The listing builds one solid part. Answer for the finished solid, in the listing's coordinates (mm). A direction names the side the tool comes from. Give positions to 0.01 mm unless a question says otherwise; leave off trailing zeros. Order: outer loops, then holes, each group sorted by start corner. A loop starts at its lowest first (then second) coordinate and runs counter-clockwise, first axis right, second up. Notation, with made-up numbers: (55.5, -5) - (96.5, -5) arc R18 cw to (96.5, 21) - close; hole circle Ø5 at (52, 1). An arc over 180 degrees is marked (long way). Answer as a JSON object with one key per item and string values. Group by question number.
Q1. The mould has two halves that part along Z. Classify faces 3 (the face through (3.71, -12.32, 66.4)), 4 (the face through (4.98, -37.57, 74.76)), 5 (the face through (6.35, -38, 40)): released by +Z, released by -Z, zero draft, split by the parting line, or undercut.
Q2. Given pin 1 (9 mm diameter, centred on y = -12.7, z = 63.5, fed in from +X); pin 2 (2 mm diameter, centred on x = 54.5, y = -38.5, fed in from +Z) (3 decimals); pin 3 (7.5 mm diameter, centred on y = -63.5, z = 63.5, fed in from -X); pin 4 (10 mm diameter, centred on y = -52, z = 24.5, fed in from +X), each flat-ended and moving along its own axis, determine where each tip first touches the part or whether it passes through.
Q3. Consider line 1 (Y direction, x = 2.5, z = 25.4); line 2 (Z direction, x = 1.05, y = -12.7); line 3 (Z direction, x = 2.9, y = -63.5). Determine where each line is inside the solid, lowest interval first.
Q4. For faces 1 (the face through (127, -38, 2)), 2 (the face through (65, -38, 9.525)), determine the directions among +Z, -Z, +X, -X, +Y, -Y from which every point of the face is accessible in a straight line to the end or side of a thin tool.
Q5. A cutting plane is placed at C-C, the plane y = -63.5. Give the vertices of the cut face in (x, z) (3 decimals).
Q6. A cutting plane is placed at D-D, the plane y = -49.5. Give the vertices of the cut face in (x, z) (3 decimals), and give its area (3 significant figures).
Q7. A cutting plane is placed at B-B, the plane z = 25.4. Give the vertices of the cut face in (x, y), and give its area (3 significant figures).
Q8. A cutting plane is placed at A-A, the plane y = -38.1. Give the vertices of the cut face in (x, z) (3 decimals), and give its area (3 significant figures).
from build123d import *

# Parameters (mm, degrees)
F1_DEPTH       = 76.2
F3_D           = 8.5
F5_D           = 5.6134
F5_CSINK_D     = 10.4394
F5_CSINK_ANGLE = 82


with BuildPart() as f1:
    # F0 (on Front) → F1 (new body)
    with BuildSketch(Plane.XZ):
        with BuildLine():
            Line((0, 76.2), (0, 0))
            Line((0, 0), (127, 0))
            Line((127, 0), (127, 4.725))
            ThreePointArc((127, 4.725), (125.5941125497, 8.1191125497), (122.2, 9.525))
            Line((122.2, 9.525), (6.35, 9.525))
            Line((6.35, 9.525), (6.35, 71.4))
            ThreePointArc((6.35, 71.4), (4.9441125497, 74.7941125497), (1.55, 76.2))
            Line((1.55, 76.2), (0, 76.2))
        make_face()
    extrude(amount=F1_DEPTH)

    # F3 (through all)
    with Locations(Plane.XY.offset(9.525)):
        with Locations((72.23125, -38.1)):
            Hole(F3_D / 2)

    # F5 (through all)
    with Locations(Plane.YZ.offset(6.35)):
        with Locations((-63.5, 63.5), (-63.5, 25.4), (-12.7, 25.4), (-12.7, 63.5)):
            CounterSinkHole(F5_D / 2, F5_CSINK_D / 2, counter_sink_angle=F5_CSINK_ANGLE)


solid = f1.part
Reply:
{
 "1": {"face 3": "undercut", "face 4": "released by +Z", "face 5": "zero draft"},
 "2": {"pin 1": "stops at x = 5.52", "pin 2": "stops at z = 9.525", "pin 3": "stops at x = 0", "pin 4": "stops at x = 6.35"},
 "3": {"line 1": "y = -76.2 to -66.31, -60.69 to -15.51, -9.89 to 0", "line 2": "z = 0 to 22.59, 28.21 to 60.69, 66.31 to 76.2", "line 3": "z = 0 to 22.59, 28.21 to 60.69, 66.31 to 76.01"},
 "4": {"face 1": "+Z, -Z, +X, +Y, -Y", "face 2": "+Z, +X, +Y, -Y"},
 "5": {"outline": "(0, 0) - (127, 0) - (127, 4.725) arc R4.8 ccw to (122.2, 9.525) - (6.35, 9.525) - (6.35, 20.18) - (3.574, 22.593) - (0, 22.593) - close; (0, 28.207) - (3.574, 28.207) - (6.35, 30.62) - (6.35, 58.28) - (3.574, 60.693) - (0, 60.693) - close; (0, 66.307) - (3.574, 66.307) - (6.35, 68.72) - (6.35, 71.4) arc R4.8 ccw to (1.55, 76.2) - (0, 76.2) - close"},
 "6": {"outline": "(0, 0) - (127, 0) - (127, 4.725) arc R4.8 ccw to (122.2, 9.525) - (6.35, 9.525) - (6.35, 71.4) arc R4.8 ccw to (1.55, 76.2) - (0, 76.2) - close", "area": "1,620 mm^2"},
 "7": {"outline": "(0, -76.2) - (6.35, -76.2) - (6.35, -68.72) - (3.57, -66.31) - (0, -66.31) - close; (0, -60.69) - (3.57, -60.69) - (6.35, -58.28) - (6.35, -17.92) - (3.57, -15.51) - (0, -15.51) - close; (0, -9.89) - (3.57, -9.89) - (6.35, -7.48) - (6.35, 0) - (0, 0) - close", "area": "399 mm^2"},
 "8": {"outline": "(0, 0) - (67.981, 0) - (67.981, 9.525) - (6.35, 9.525) - (6.35, 71.4) arc R4.8 ccw to (1.55, 76.2) - (0, 76.2) - close; (76.481, 0) - (127, 0) - (127, 4.725) arc R4.8 ccw to (122.2, 9.525) - (76.481, 9.525) - close", "area": "1,540 mm^2"}
}
